The model under review builds one solid part; all positions refer to its coordinate system, in mm. Face numbers are marked on the shaded views. A direction names the side the tool comes from. Coordinates: 2 decimals unless noted, no trailing zeros. Order: outer loops, then holes, each group sorted by start corner. A loop starts at its lowest first (then second) coordinate and runs counter-clockwise, first axis right, second up. Notation, with made-up numbers: M 25.5,53 L 76.5,53 A25 ccw 76.5,89 Z; hole C -24,45.25 d6. An arc over 180 degrees is marked long. Answer as CSV lines item,"result". Start each with the question number.
Q1. Consider section A-A on z = 23.75. Write out the cut boundary in (x, y) (3 decimals), and give its area (3 significant figures).
Q2. Consider section D-D on z = 17.5. Write out the cut boundary in (x, y) (3 decimals).
Q3. Machinability: for the marked faces 4 and 5, which of the approach directions +Z, -Z, +X, -X, +Y, -Y give a long, thin tool a straight path to every point of the face, cutting with its end or side? Answer none if there is none.
Q4. Wall thickness on L1, parallel to Y at x = 0, z = 23.65; L2, parallel to Y at x = 0, z = 14.25; L3, parallel to X at y = 3, z = 20.75: over which ranges is each line inside the solid? List them lowest first. Write a range as [from, to].
Q5. The part is to be moulded in two halves that separate along X. For the marked faces 1, 2 and 3, say which applies: +X half, -X half, draft (parallel to the pull), parting line (faces both ways), or undercut.
Q6. Consider section C-C on y = 0. Write out the cut boundary in (x, z), and give its area (3 significant figures).
Q7. For P1, Ø0.5, axis at y = 8, z = 17.5, coming from the -X side; P2, Ø6, axis at y = 4, z = 13, coming from the -X side; P3, Ø9.5, axis at x = 0, y = 0, coming from the -Z side; P4, Ø8, axis at y = -9, z = 13.5, coming from the -X side (3 decimals), all flat-tipped, find the tip position at first contact; note any pin that passes through.
Q8. Consider section B-B on x = 0. Write out the cut boundary in (y, z), and give its area (3 significant figures).
from build123d import *

# Parameters (mm, degrees)
SKETCH1_R           = 8.509
SKETCH1_R_2         = 5.334
BOSS_EXTRUDE1_DEPTH = 25.4
SKETCH2_R           = 7.747
SKETCH2_R_2         = 6.731
CUT_EXTRUDE1_DEPTH  = 5.08
BOSS_EXTRUDE2_DEPTH = 25.4


with BuildPart() as part:
    # Sketch1 → Boss-Extrude1 (new body)
    with BuildSketch(Plane.XY):
        Circle(SKETCH1_R)
        Circle(SKETCH1_R_2, mode=Mode.SUBTRACT)
    extrude(amount=BOSS_EXTRUDE1_DEPTH)

    # Sketch2 → Cut-Extrude1 (cut)
    with BuildSketch(Plane.XY.offset(25.4)):
        Circle(SKETCH2_R)
        Circle(SKETCH2_R_2, mode=Mode.SUBTRACT)
    extrude(amount=-CUT_EXTRUDE1_DEPTH, mode=Mode.SUBTRACT)

    # Sketch3 → Boss-Extrude2 (add)
    with BuildSketch(Plane.XY):
        with BuildLine():
            Line((-3.175, 7.894457296), (-3.175, 8.509))
            Line((-3.175, 8.509), (-4.641469684, 11.049))
            Line((-4.641469684, 11.049), (4.641469684, 11.049))
            Line((4.641469684, 11.049), (3.175, 8.509))
            Line((3.175, 8.509), (3.175, 7.894457296))
            ThreePointArc((3.175, 7.894457296), (0, 8.509), (-3.175, 7.894457296))
        make_face()
    boss_extrude2 = extrude(amount=BOSS_EXTRUDE2_DEPTH)

    # Mirror1: Boss-Extrude2 across plane
    add(boss_extrude2.mirror(Plane.ZX))


solid = part.part
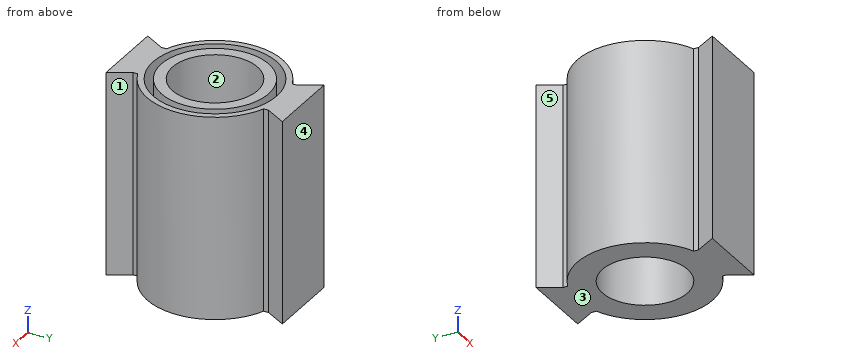
Evaluation:
1,outline,"C 0,0 d13.462; M -4.641,-11.049 L 4.641,-11.049 L 3.175,-8.509 L 3.175,-7.894 A8.509 ccw 3.175,7.894 L 3.175,8.509 L 4.641,11.049 L -4.641,11.049 L -3.175,8.509 L -3.175,7.894 A8.509 ccw -3.175,-7.894 L -3.175,-8.509 Z; hole C 0,0 d15.494; hole C 0,0 d10.668"
1,area,"134 mm²"
2,outline,"M -4.641,-11.049 L 4.641,-11.049 L 3.175,-8.509 L 3.175,-7.894 A8.509 ccw 3.175,7.894 L 3.175,8.509 L 4.641,11.049 L -4.641,11.049 L -3.175,8.509 L -3.175,7.894 A8.509 ccw -3.175,-7.894 L -3.175,-8.509 Z; hole C 0,0 d10.668"
3,face 4,"+Z, -Z, +X, -X, +Y"
3,face 5,"+Z, -Z, -X"
4,L1,"y = [-11.05, -7.75], [-6.73, -5.33], [5.33, 6.73], [7.75, 11.05]"
4,L2,"y = [-11.05, -5.33], [5.33, 11.05]"
4,L3,"x = [-7.96, -7.14], [-6.03, -4.41], [4.41, 6.03], [7.14, 7.96]"
5,face 1,"+X half"
5,face 2,"undercut"
5,face 3,"draft"
6,outline,"M -8.51,0 L -5.33,0 L -5.33,25.4 L -6.73,25.4 L -6.73,20.32 L -7.75,20.32 L -7.75,25.4 L -8.51,25.4 Z; M 5.33,0 L 8.51,0 L 8.51,25.4 L 7.75,25.4 L 7.75,20.32 L 6.73,20.32 L 6.73,25.4 L 5.33,25.4 Z"
6,area,"151 mm²"
7,P1,"stops at x = -3.51"
7,P2,"stops at x = -8.45"
7,P3,"passes through"
7,P4,"stops at x = -6.885"
8,outline,"M -11.05,0 L -5.33,0 L -5.33,25.4 L -6.73,25.4 L -6.73,20.32 L -7.75,20.32 L -7.75,25.4 L -11.05,25.4 Z; M 5.33,0 L 11.05,0 L 11.05,25.4 L 7.75,25.4 L 7.75,20.32 L 6.73,20.32 L 6.73,25.4 L 5.33,25.4 Z"
8,area,"280 mm²"
